Part model, mm, in its own coordinate system. Face numbers are marked on the shaded views. A direction names the side the tool comes from. Coordinates: 2 decimals unless noted, no trailing zeros. Loops run counter-clockwise (first coordinate to the right, second up) from the corner with the lowest first, then second, coordinate; pieces in that order, holes last. Notation, with made-up numbers: (-6, 26.25) - (26, 26.25) arc R23 cw to (26, 35.25) - close; hole circle Ø11 at (66.25, 21.5). An arc over 180 degrees is marked (long way). Use a Markdown table: item, result. Add a question column.
1) Tool access for the marked faces 5, 6 and 7: list every direction of +Z, -Z, +X, -X, +Y, -Y with a clear straight run to the whole face (end or side of a thin tool).
2) Pull direction Y, two halves, no side cores. Call the marked faces 1, 2, 3 and 4: +Y half, -Y half, draft (parallel to the pull), parting line (faces both ways), or undercut.
3) Band-saw the part on B-B (y = 95). Give the cut face in (x, z).
4) Drop flat-ended pins along their axis: P1, Ø1.5, axis at y = 15, z = 38, coming from the -X side; P2, Ø12, axis at y = 25, z = 55, coming from the -X side; P3, Ø3, axis at y = 50, z = 51.5, coming from the -X side; P4, Ø6, axis at x = 103, z = 54, coming from the -Y side. Give the stop position or say it passes through.
5) Probe probe 1 along Y at (x, z) = (105, 22); probe 2 along Y at (x, z) = (105, 42.5); probe 3 along Z at (x, y) = (138, 25). List the from-to ranges inside material, lowest first. Write a range as [from, to].
6) Band-saw the part on A-A (z = 55). Give the cut face in (x, y), plus the area to 3 significant figures.
7) Band-saw the part on C-C (x = 105). Give the cut face in (y, z).
8) Band-saw the part on D-D (z = 43). Give the cut face in (x, y).
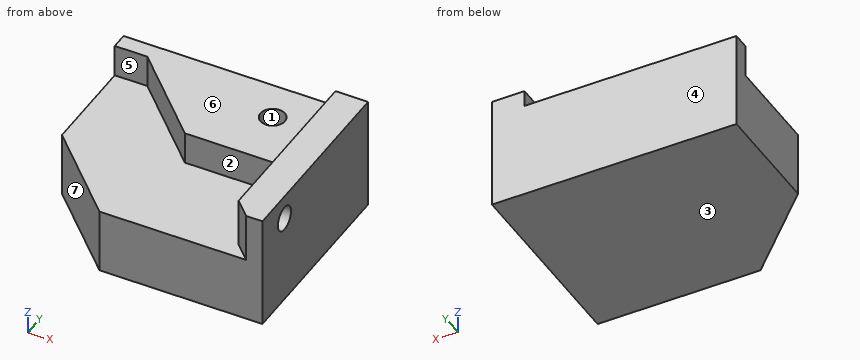
Autodesk Fusion 360 part; units mm, degrees
sketch "Sketch1" plane through (0, 0, 0) normal (0, 0, 1) x (1, 0, 0)
  line L0 (50, 0) -> (150, 0)
  line L1 (150, 0) -> (150, 120)
  line L2 (150, 120) -> (0, 120)
  line L3 (0, 120) -> (0, 50)
  line L4 (0, 50) -> (50, 0)
  line L5 (0, 50) -> (0, 0)
  line L6 (0, 0) -> (50, 0)
  line L7 (0, 110) -> (20, 110)
  line L8 (20, 110) -> (70, 60)
  line L9 (70, 60) -> (130, 60)
  line L10 (130, 60) -> (130, 120)
  line L11 (130, 60) -> (130, 10)
  line L12 (130, 10) -> (140, 0)
  dimension "d2" = 120
  dimension "d3" = 50
  dimension "d4" = 135
  dimension "d5" = 10
  dimension "d6" = 10
  dimension "d7" = 10
  dimension "d8" = 60
  dimension "d9" = 135
  dimension "d10" = 20
  dimension "d17" = 60
extrude "Extrude1" add sketch "Sketch1" along normal blind 40 contours L0 L3 L4 L7 L8 L9 L11 L12
extrude "Extrude2" add sketch "Sketch1" along normal blind 60 contours L2 L3 L7 L8 L9 L10
extrude "Extrude3" add sketch "Sketch1" along normal blind 70 contours L0 L1 L2 L10 L11 L12
sketch "Sketch2" plane through (0, 0, 60) normal (0, 0, 1) x (-1, 0, 0)
  line L0 (-130, -60) -> (-130, -120)
  line L1 (-130, -120) -> (0, -120)
  line L2 (0, -120) -> (0, -110)
  line L3 (0, -110) -> (-20, -110)
  line L4 (-20, -110) -> (-70, -60)
  line L5 (-70, -60) -> (-130, -60)
  circle A0 centre (-105, -95) radius 7.5
  dimension "d23" = 15
  dimension "d24" = 25
  dimension "d25" = 25
sketch "Sketch3" plane through (130, 0, 0) normal (-1, 0, 0) x (0, -1, 0)
  line L0 (-60, 40) -> (-10, 40)
  line L1 (-10, 40) -> (-10, 70)
  line L2 (-10, 70) -> (-120, 70)
  line L3 (-60, 60) -> (-60, 40)
  circle A0 centre (-25, 55) radius 7.5
  line L4 (-120, 70) -> (-120, 60)
  line L5 (-120, 60) -> (-60, 60)
  dimension "d26" = 15
  dimension "d27" = 15
  dimension "d28" = 15
extrude "Extrude4" cut sketch "Sketch3" against normal blind 30 contours A0
extrude "Extrude5" cut sketch "Sketch2" against normal blind 50 contours A0
Answer block:
| question | item | result |
|---|---|---|
| 1 | face 5 | +Z, -X, -Y |
| 1 | face 6 | +Z, -X, +Y, -Y |
| 1 | face 7 | +Z, -Z, -X, -Y |
| 2 | face 1 | undercut |
| 2 | face 2 | -Y half |
| 2 | face 3 | draft |
| 2 | face 4 | +Y half |
| 3 | outline | (0, 0) - (150, 0) - (150, 70) - (130, 70) - (130, 60) - (112.5, 60) - (112.5, 10) - (97.5, 10) - (97.5, 60) - (35, 60) - (35, 40) - (0, 40) - close |
| 4 | P1 | x = 34.25 |
| 4 | P2 | through |
| 4 | P3 | x = 130 |
| 4 | P4 | y = 60 |
| 5 | probe 1 | [0, 87.5], [102.5, 120] |
| 5 | probe 2 | [60, 87.5], [102.5, 120] |
| 5 | probe 3 | [0, 47.5], [62.5, 70] |
| 6 | outline | (0, 110) - (20, 110) - (70, 60) - (130, 60) - (130, 32.5) - (150, 32.5) - (150, 120) - (0, 120) - close; (130, 10) - (140, 0) - (150, 0) - (150, 17.5) - (130, 17.5) - close; hole circle Ø15 at (105, 95) |
| 6 | area | 7,420 mm2 |
| 7 | outline | (0, 0) - (120, 0) - (120, 60) - (102.5, 60) - (102.5, 10) - (87.5, 10) - (87.5, 60) - (60, 60) - (60, 40) - (0, 40) - close |
| 8 | outline | (0, 110) - (20, 110) - (70, 60) - (130, 60) - (130, 10) - (140, 0) - (150, 0) - (150, 120) - (0, 120) - close; hole circle Ø15 at (105, 95) |
